```python
from build123d import *

# Parameters (mm, degrees)
SKETCH1_R           = 1.6383
SKETCH1_R_2         = 0.8382
BOSS_EXTRUDE1_DEPTH = 1.575
CUT_EXTRUDE1_DEPTH  = 2.54
SKETCH15_R          = 0.8382
CUT_EXTRUDE5_DEPTH  = 1.575
BOSS_EXTRUDE2_DEPTH = 1.575


with BuildPart() as part:
    # Sketch1 → Boss-Extrude1 (new body)
    with BuildSketch(Plane(origin=(0, 0, 0), x_dir=(1, 0, 0), z_dir=(0, 1, 0))):
        with BuildLine():
            Line((-44, 45), (-44, 30.998648377))
            ThreePointArc((-44, 30.998648377), (-43.707106781, 30.291541596), (-43, 29.998648377))
            Line((-43, 29.998648377), (-33.824, 29.998648377))
            ThreePointArc((-33.824, 29.998648377), (-33.116893219, 29.705755158), (-32.824, 28.998648377))
            Line((-32.824, 28.998648377), (-32.824, -30.469351623))
            ThreePointArc((-32.824, -30.469351623), (-33.116893219, -31.176458404), (-33.824, -31.469351623))
            Line((-33.824, -31.469351623), (-36.100000052, -31.469351623))
            Line((-36.100000052, -31.469351623), (-42.999999948, -31.469351623))
            ThreePointArc((-42.999999948, -31.469351623), (-43.707106729, -31.762244842), (-43.999999948, -32.469351623))
            Line((-43.999999948, -32.469351623), (-43.999999948, -38.977))
            Line((-43.999999948, -38.977), (-43.999999948, -45))
            ThreePointArc((-43.999999948, -45), (-43.41421351, -46.414213562), (-41.999999948, -47))
            Line((-41.999999948, -47), (42.705916546, -47))
            Line((42.705916546, -47), (43.849731117, -47))
            Line((43.849731117, -47), (43.849731117, -38.27))
            Line((43.849731117, -38.27), (43.849731117, -32.469351623))
            ThreePointArc((43.849731117, -32.469351623), (43.556837899, -31.762244842), (42.849731117, -31.469351623))
            Line((42.849731117, -31.469351623), (36.100000052, -31.469351623))
            Line((36.100000052, -31.469351623), (33.824, -31.469351623))
            ThreePointArc((33.824, -31.469351623), (33.116893219, -31.176458404), (32.824, -30.469351623))
            Line((32.824, -30.469351623), (32.824, 28.998648377))
            ThreePointArc((32.824, 28.998648377), (33.116893219, 29.705755158), (33.824, 29.998648377))
            Line((33.824, 29.998648377), (43, 29.998648377))
            ThreePointArc((43, 29.998648377), (43.707106781, 30.291541596), (44, 30.998648377))
            Line((44, 30.998648377), (44, 31.284))
            Line((44, 31.284), (44, 45))
            ThreePointArc((44, 45), (43.414213562, 46.414213562), (42, 47))
            Line((42, 47), (-42, 47))
            ThreePointArc((-42, 47), (-43.414213562, 46.414213562), (-44, 45))
        make_face()
        with Locations(Location((40, 43.5, 0), (0, 0, 270))):
            Circle(SKETCH1_R, mode=Mode.SUBTRACT)
        with Locations(Location((-40, 43.5, 0), (0, 0, 270))):
            Circle(SKETCH1_R, mode=Mode.SUBTRACT)
        with Locations(Location((-37.599999948, -42.2, 0), (0, 0, 270))):
            Circle(SKETCH1_R, mode=Mode.SUBTRACT)
        with Locations(Location((36.100000052, -42.2, 0), (0, 0, 270))):
            Circle(SKETCH1_R, mode=Mode.SUBTRACT)
        with Locations(Location((26.22, 17.931928709, 0), (0, 0, 270))):
            Circle(SKETCH1_R_2, mode=Mode.SUBTRACT)
        with Locations(Location((-26.22, 17.931928709, 0), (0, 0, 270))):
            Circle(SKETCH1_R_2, mode=Mode.SUBTRACT)
        Polygon((23.409, -31.5), (-23.409, -31.5), (-23.409, 13.29544), (-12.909, 13.29544), (-12.909, 25.99544), (12.909, 25.99544), (12.909, 13.29544), (23.409, 13.29544), align=None, mode=Mode.SUBTRACT)
    extrude(amount=BOSS_EXTRUDE1_DEPTH)

    # Sketch2 → Cut-Extrude1 (cut)
    with BuildSketch(Plane(origin=(0, 1.575, 0), x_dir=(1, 0, 0), z_dir=(0, 1, 0))):
        Polygon((-12.909, 19.06), (-30.435, 19.06), (-30.435, 47), (30.435, 47), (30.435, 19.06), (12.909, 19.06), (12.909, 25.99544), (-12.909, 25.99544), align=None)
    extrude(amount=-CUT_EXTRUDE1_DEPTH, mode=Mode.SUBTRACT)

    # Sketch15 → Cut-Extrude5 (cut)
    with BuildSketch(Plane(origin=(0, 1.575, 0), x_dir=(1, 0, 0), z_dir=(0, 1, 0))):
        with Locations(Location((-36.785, 36.35, 0), (0, 0, 270))):
            Circle(SKETCH15_R)
        with Locations(Location((36.785, 36.332, 0), (0, 0, 270))):
            Circle(SKETCH15_R)
    extrude(amount=-CUT_EXTRUDE5_DEPTH, mode=Mode.SUBTRACT)

    # Sketch16 → Boss-Extrude2 (add)
    with BuildSketch(Plane(origin=(0, 1.575, 0), x_dir=(1, 0, 0), z_dir=(0, 1, 0))):
        Polygon((12.909, 19.06), (12.909, 13.29544), (-12.909, 13.29544), (-12.909, 19.06), (-30.435, 19.06), (-30.435, 22.25535429), (-11.909, 22.25535429), (-11.909, 47), (11.909, 47), (11.909, 22.25535429), (30.435, 22.25535429), (30.435, 19.06), align=None)
    extrude(amount=-BOSS_EXTRUDE2_DEPTH)


solid = part.part
```
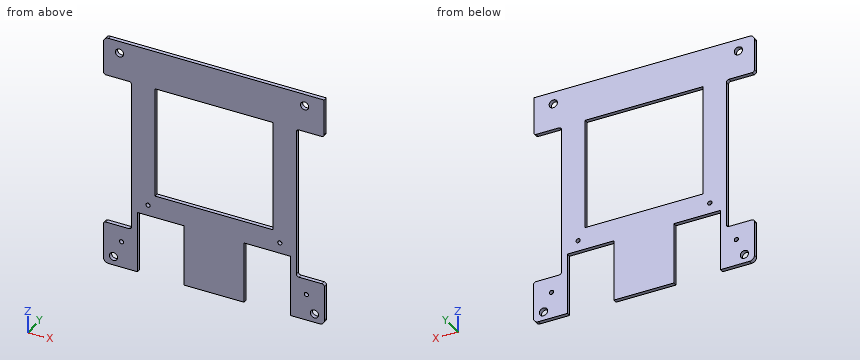
The listing builds one solid part. Answer for the finished solid, in the listing's coordinates (mm). Round coordinates to 2 decimals unless told otherwise and drop trailing zeros. Write each loop counter-clockwise with the first axis right and the second up, starting at its lowest first coordinate (ties: lowest second). Pieces come first, ordered by that corner, then holes. Notation, with made-up numbers: (-0.75, -2) -> (58.25, -2) arc R24 cw to (58.25, 21) -> close; hole circle Ø9 at (-39.75, -28.5). An arc over 180 degrees is marked (long way). Use CSV: the item, a comma, the result in double quotes. Start each with the question number.
(1) Consider L1, parallel to X at y = 0.95, z = 42.2; L2, parallel to X at y = 0.95, z = -43.5 (3 decimals); L3, parallel to X at y = 0.15, z = -39 (3 decimals). Determine where each line is inside the solid, lowest interval first. Write a range as from..to.
(2) Section A-A on x = -1 is taken. Give the vertices of the cut face in (y, z) (3 decimals).
(3) Section B-B on z = -43.5 is taken. Give the vertices of the cut face in (x, y) (3 decimals), then the cut area to 3 significant figures.
(4) Section D-D on z = -15.5 is taken. Give the vertices of the cut face in (x, y) (3 decimals).
(5) Each of these flat-tipped pins is pushed along its axis until it touches: pin 1 (8 mm diameter, centred on x = 35, z = 2.5, fed in from -Y); pin 2 (0.5 mm diameter, centred on y = 1, z = -29.5, fed in from +X). Where does it stop, or does it pass through?
(6) Section C-C on z = 27 is taken. Give the vertices of the cut face in (x, y) (3 decimals), then the cut area to 3 significant figures.
A:
1,L1,"x = -44..-39.24, -35.96..34.46, 37.74..43.85"
1,L2,"x = -44..-41.638, -38.362..-30.435, -11.909..11.909, 30.435..38.362, 41.638..44"
1,L3,"x = -44..-30.435, -11.909..11.909, 30.435..44"
2,outline,"(0, -47) -> (1.575, -47) -> (1.575, -13.295) -> (0, -13.295) -> close; (0, 31.5) -> (1.575, 31.5) -> (1.575, 47) -> (0, 47) -> close"
3,outline,"(-44, 0) -> (-41.638, 0) -> (-41.638, 1.575) -> (-44, 1.575) -> close; (-38.362, 0) -> (-30.435, 0) -> (-30.435, 1.575) -> (-38.362, 1.575) -> close; (-11.909, 0) -> (11.909, 0) -> (11.909, 1.575) -> (-11.909, 1.575) -> close; (30.435, 0) -> (38.362, 0) -> (38.362, 1.575) -> (30.435, 1.575) -> close; (41.638, 0) -> (44, 0) -> (44, 1.575) -> (41.638, 1.575) -> close"
3,area,"69.9 mm²"
4,outline,"(-32.824, 0) -> (32.824, 0) -> (32.824, 1.575) -> (-32.824, 1.575) -> close"
5,pin 1,"stops at y = 0"
5,pin 2,"stops at x = 33.16"
6,outline,"(-32.824, 0) -> (-23.409, 0) -> (-23.409, 1.575) -> (-32.824, 1.575) -> close; (23.409, 0) -> (32.824, 0) -> (32.824, 1.575) -> (23.409, 1.575) -> close"
6,area,"29.7 mm²"
